Model file for the job. Use its own axes, mm. A direction names the side the tool comes from. Round coordinates to 2 decimals unless told otherwise and drop trailing zeros. Loops run counter-clockwise (first coordinate to the right, second up) from the corner with the lowest first, then second, coordinate; pieces in that order, holes last. Notation, with made-up numbers: (-12.5, 50) - (28.5, 50) arc R29 cw to (28.5, 85) - close; hole circle Ø9 at (54.25, 68.5). An arc over 180 degrees is marked (long way). Answer as a JSON object with one key per item and string values.
from build123d import *

# Parameters (mm, degrees)
AUFSATZ_LINEAR_AUSTRAGEN2_DEPTH = 2
SCHNITT_LINEAR_AUSTRAGEN2_DEPTH = 2


with BuildPart() as part:
    # Skizze2 → Aufsatz-Linear austragen2 (new body)
    with BuildSketch(Plane(origin=(0, 0, 0), x_dir=(1, 0, 0), z_dir=(0, 1, 0))):
        with BuildLine():
            Line((-44, 50), (-28, 50))
            Line((-28, 50), (-16.61985221, 33))
            ThreePointArc((-16.61985221, 33), (0, 24.125669082), (16.61985221, 33))
            Line((16.61985221, 33), (28, 50))
            Line((28, 50), (44, 50))
            ThreePointArc((44, 50), (47.535533906, 48.535533906), (49, 45))
            Line((49, 45), (49, -49))
            Line((49, -49), (-49, -49))
            Line((-49, -49), (-49, 45))
            ThreePointArc((-49, 45), (-47.535533906, 48.535533906), (-44, 50))
        make_face()
    extrude(amount=AUFSATZ_LINEAR_AUSTRAGEN2_DEPTH)

    # Skizze3 → Schnitt-Linear austragen2 (cut)
    with BuildSketch(Plane(origin=(0, 2, 0), x_dir=(1, 0, 0), z_dir=(0, 1, 0))):
        with BuildLine():
            Line((-39.25, 15), (-5.75, 15))
            ThreePointArc((-5.75, 15), (-4.335786438, 14.414213562), (-3.75, 13))
            Line((-3.75, 13), (-3.75, 9))
            ThreePointArc((-3.75, 9), (-4.335786438, 7.585786438), (-5.75, 7))
            Line((-5.75, 7), (-39.25, 7))
            ThreePointArc((-39.25, 7), (-40.664213562, 7.585786438), (-41.25, 9))
            Line((-41.25, 9), (-41.25, 13))
            ThreePointArc((-41.25, 13), (-40.664213562, 14.414213562), (-39.25, 15))
        make_face()
        with BuildLine():
            Line((3.75, 13), (3.75, 9))
            ThreePointArc((3.75, 9), (4.335786438, 7.585786438), (5.75, 7))
            Line((5.75, 7), (39.25, 7))
            ThreePointArc((39.25, 7), (40.664213562, 7.585786438), (41.25, 9))
            Line((41.25, 9), (41.25, 13))
            ThreePointArc((41.25, 13), (40.664213562, 14.414213562), (39.25, 15))
            Line((39.25, 15), (5.75, 15))
            ThreePointArc((5.75, 15), (4.335786438, 14.414213562), (3.75, 13))
        make_face()
        with BuildLine():
            Line((3.75, 1), (3.75, -3))
            ThreePointArc((3.75, -3), (4.335786438, -4.414213562), (5.75, -5))
            Line((5.75, -5), (39.25, -5))
            ThreePointArc((39.25, -5), (40.664213562, -4.414213562), (41.25, -3))
            Line((41.25, -3), (41.25, 1))
            ThreePointArc((41.25, 1), (40.664213562, 2.414213562), (39.25, 3))
            Line((39.25, 3), (5.75, 3))
            ThreePointArc((5.75, 3), (4.335786438, 2.414213562), (3.75, 1))
        make_face()
        with BuildLine():
            Line((3.75, -11), (3.75, -15))
            ThreePointArc((3.75, -15), (4.335786438, -16.414213562), (5.75, -17))
            Line((5.75, -17), (39.25, -17))
            ThreePointArc((39.25, -17), (40.664213562, -16.414213562), (41.25, -15))
            Line((41.25, -15), (41.25, -11))
            ThreePointArc((41.25, -11), (40.664213562, -9.585786438), (39.25, -9))
            Line((39.25, -9), (5.75, -9))
            ThreePointArc((5.75, -9), (4.335786438, -9.585786438), (3.75, -11))
        make_face()
        with BuildLine():
            Line((3.75, -23), (3.75, -27))
            ThreePointArc((3.75, -27), (4.335786438, -28.414213562), (5.75, -29))
            Line((5.75, -29), (39.25, -29))
            ThreePointArc((39.25, -29), (40.664213562, -28.414213562), (41.25, -27))
            Line((41.25, -27), (41.25, -23))
            ThreePointArc((41.25, -23), (40.664213562, -21.585786438), (39.25, -21))
            Line((39.25, -21), (5.75, -21))
            ThreePointArc((5.75, -21), (4.335786438, -21.585786438), (3.75, -23))
        make_face()
        with BuildLine():
            Line((3.75, -35), (3.75, -39))
            ThreePointArc((3.75, -39), (4.335786438, -40.414213562), (5.75, -41))
            Line((5.75, -41), (39.25, -41))
            ThreePointArc((39.25, -41), (40.664213562, -40.414213562), (41.25, -39))
            Line((41.25, -39), (41.25, -35))
            ThreePointArc((41.25, -35), (40.664213562, -33.585786438), (39.25, -33))
            Line((39.25, -33), (5.75, -33))
            ThreePointArc((5.75, -33), (4.335786438, -33.585786438), (3.75, -35))
        make_face()
        with BuildLine():
            Line((-41.25, 1), (-41.25, -3))
            ThreePointArc((-41.25, -3), (-40.664213562, -4.414213562), (-39.25, -5))
            Line((-39.25, -5), (-5.75, -5))
            ThreePointArc((-5.75, -5), (-4.335786438, -4.414213562), (-3.75, -3))
            Line((-3.75, -3), (-3.75, 1))
            ThreePointArc((-3.75, 1), (-4.335786438, 2.414213562), (-5.75, 3))
            Line((-5.75, 3), (-39.25, 3))
            ThreePointArc((-39.25, 3), (-40.664213562, 2.414213562), (-41.25, 1))
        make_face()
        with BuildLine():
            Line((-41.25, -11), (-41.25, -15))
            ThreePointArc((-41.25, -15), (-40.664213562, -16.414213562), (-39.25, -17))
            Line((-39.25, -17), (-5.75, -17))
            ThreePointArc((-5.75, -17), (-4.335786438, -16.414213562), (-3.75, -15))
            Line((-3.75, -15), (-3.75, -11))
            ThreePointArc((-3.75, -11), (-4.335786438, -9.585786438), (-5.75, -9))
            Line((-5.75, -9), (-39.25, -9))
            ThreePointArc((-39.25, -9), (-40.664213562, -9.585786438), (-41.25, -11))
        make_face()
        with BuildLine():
            Line((-41.25, -23), (-41.25, -27))
            ThreePointArc((-41.25, -27), (-40.664213562, -28.414213562), (-39.25, -29))
            Line((-39.25, -29), (-5.75, -29))
            ThreePointArc((-5.75, -29), (-4.335786438, -28.414213562), (-3.75, -27))
            Line((-3.75, -27), (-3.75, -23))
            ThreePointArc((-3.75, -23), (-4.335786438, -21.585786438), (-5.75, -21))
            Line((-5.75, -21), (-39.25, -21))
            ThreePointArc((-39.25, -21), (-40.664213562, -21.585786438), (-41.25, -23))
        make_face()
        with BuildLine():
            Line((-41.25, -35), (-41.25, -39))
            ThreePointArc((-41.25, -39), (-40.664213562, -40.414213562), (-39.25, -41))
            Line((-39.25, -41), (-5.75, -41))
            ThreePointArc((-5.75, -41), (-4.335786438, -40.414213562), (-3.75, -39))
            Line((-3.75, -39), (-3.75, -35))
            ThreePointArc((-3.75, -35), (-4.335786438, -33.585786438), (-5.75, -33))
            Line((-5.75, -33), (-39.25, -33))
            ThreePointArc((-39.25, -33), (-40.664213562, -33.585786438), (-41.25, -35))
        make_face()
    extrude(amount=-SCHNITT_LINEAR_AUSTRAGEN2_DEPTH, mode=Mode.SUBTRACT)


solid = part.part
1) Slice it at D-D on x = 21.5. List the corners of the cut face in (y, z).
Values follow:
{"outline": "(0, -40.29) - (2, -40.29) - (2, -15) - (0, -15) - close; (0, -7) - (2, -7) - (2, -3) - (0, -3) - close; (0, 5) - (2, 5) - (2, 9) - (0, 9) - close; (0, 17) - (2, 17) - (2, 21) - (0, 21) - close; (0, 29) - (2, 29) - (2, 33) - (0, 33) - close; (0, 41) - (2, 41) - (2, 49) - (0, 49) - close"}
2) Slice it at C-C on y = 1.1. Count the separate pieces of the cut face and the enclosed holes in it, then the cut area to 3 significant figures.
Values follow:
{"separate pieces": "1", "enclosed holes": "10", "area": "5,760 mm²"}
3) Probe probe 1 along Z at (x, y) = (28, 1.05); probe 2 along Z at (x, y) = (27, 1.15); probe 3 along X at (y, z) = (0.3, 3). List the from-to ranges inside material, lowest first.
Values follow:
{"probe 1": "-50 to -15, -7 to -3, 5 to 9, 17 to 21, 29 to 33, 41 to 49", "probe 2": "-48.51 to -15, -7 to -3, 5 to 9, 17 to 21, 29 to 33, 41 to 49", "probe 3": "-49 to -41.25, -3.75 to 3.75, 41.25 to 49"}
4) Tool access for faces 1 (the cylindrical face through (-48, 1, -48)), 2 (the flat face through (-22.39, 0.99, -41.62)): list every direction of +Z, -Z, +X, -X, +Y, -Y with a clear straight run to the whole face (end or side of a thin tool).
Values follow:
{"face 1": "-Z, -X, +Y, -Y", "face 2": "-Z, +Y, -Y"}
5) Two-plate mould, pull along X, no slides. Class faces 3 (the flat face through (22.23, 0.99, -41.38)), 4 (the cylindrical face through (47, 1, -49)), 5 (the flat face through (1, 0, 10)): pulls with the +X half, pulls with the -X half, needs draft (parallel to the pull), parting line crosses it, or undercut.
Values follow:
{"face 3": "undercut", "face 4": "pulls with the +X half", "face 5": "needs draft"}
6) Slice it at A-A on x = 36. List the corners of the cut face in (y, z).
Values follow:
{"outline": "(0, -50) - (2, -50) - (2, -15) - (0, -15) - close; (0, -7) - (2, -7) - (2, -3) - (0, -3) - close; (0, 5) - (2, 5) - (2, 9) - (0, 9) - close; (0, 17) - (2, 17) - (2, 21) - (0, 21) - close; (0, 29) - (2, 29) - (2, 33) - (0, 33) - close; (0, 41) - (2, 41) - (2, 49) - (0, 49) - close"}
7) Slice it at B-B on z = -29. List the corners of the cut face in (x, y).
Values follow:
{"outline": "(-49, 0) - (-13.08, 0) - (-13.08, 2) - (-49, 2) - close; (13.08, 0) - (49, 0) - (49, 2) - (13.08, 2) - close"}
8) Drop flat-ended pins along their axis: P1, Ø1, axis at x = 27, y = 1.5, coming from the -Z side; P2, Ø1, axis at x = 20.5, y = 1.5, coming from the -Z side. Give the stop position or say it passes through.
Values follow:
{"P1": "z = -49.25", "P2": "z = -39.54"}
